Work out the finished part from the listing and answer in its coordinate system (mm). Face numbers are marked on the shaded views. A direction names the side the tool comes from. Give positions to 0.01 mm unless a question says otherwise; leave off trailing zeros. Loops run counter-clockwise (first coordinate to the right, second up) from the corner with the lowest first, then second, coordinate; pieces in that order, holes last. Notation, with made-up numbers: M 41,86 L 100,86 A19 ccw 100,102 Z; hole C 33.25,63 d8. An arc over 180 degrees is marked long. Use a Markdown table: item, result.
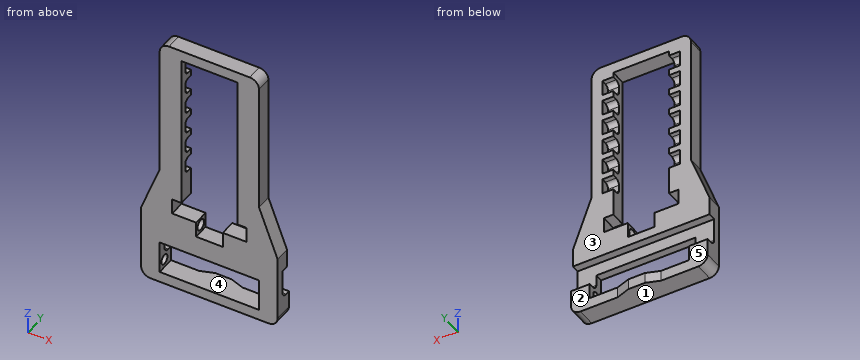
```python
from build123d import *
from OCP.BRepFilletAPI import BRepFilletAPI_MakeChamfer

# Parameters (mm, degrees)
SKETCH1_W                = 44
SKETCH1_H                = 22
BOSS_EXTRUDE1_DEPTH      = 5
SKETCH2_W                = 3.531949687
SKETCH2_H                = 41.5
SKETCH2_W_2              = 3.5
BOSS_EXTRUDE2_DEPTH      = 2
SKETCH3_W                = 44
SKETCH3_H                = 9.5
CUT_EXTRUDE1_DEPTH       = 2.5
SKETCH4_W                = 17.968050313
SKETCH4_H                = 14
CUT_EXTRUDE2_DEPTH       = 5
SKETCH5_W                = 24
SKETCH5_H                = 5
CUT_EXTRUDE3_DEPTH       = 5
SKETCH6_W                = 8.6
SKETCH6_H                = 5
CUT_EXTRUDE4_DEPTH       = 5
SKETCH7_W                = 14
SKETCH7_H                = 2
BOSS_EXTRUDE3_DEPTH      = 1.5
CHAMFER1_SIZE            = 1.5
CHAMFER1_SIZE_2          = 4.356316317
SKETCH8_W                = 32
SKETCH8_H                = 10
CUT_EXTRUDE5_DEPTH       = 5
FILLET3_R                = 3
SKETCH9_R                = 1.75
CUT_EXTRUDE6_DEPTH       = 3
CUT_EXTRUDE7_START       = -3
SKETCH10_R               = 1.75
CUT_EXTRUDE7_DEPTH       = 3
SKETCH11_R               = 1.6
CUT_EXTRUDE8_DEPTH       = 3
CUT_EXTRUDE9_START       = -3
SKETCH12_R               = 1.6
CUT_EXTRUDE9_DEPTH       = 3
SKETCH13_W               = 3.531949687
SKETCH13_H               = 2
BOSS_EXTRUDE5_DEPTH      = 3
FILLET4_R                = 1.5
BOSS_EXTRUDE6_DEPTH      = 2
BOSS_EXTRUDE6_DEPTH_BACK = 2
SKETCH15_W               = 6
SKETCH15_H               = 1
BOSS_EXTRUDE7_DEPTH      = 4.5
FILLET5_R                = 2
FILLET6_R                = 3
CUT_EXTRUDE10_DEPTH      = 14.5
CUT_EXTRUDE10_DEPTH_BACK = 14.5
SKETCH16_W               = 32
SKETCH16_H               = 0.5


with BuildPart() as part:
    # Sketch1 → Boss-Extrude1 (new body)
    with BuildSketch(Plane(origin=(0, 0, 0), x_dir=(1, 0, 0), z_dir=(0, 1, 0))):
        with Locations((0, 9)):
            Rectangle(SKETCH1_W, SKETCH1_H)
        Polygon((-16, -18), (16, -18), (22, -2), (-22, -2), align=None)
        Polygon((-12.5, -18), (-16, -18), (-16, -63), (16, -63), (16, -18), (12.5, -18), (12.5, -59.5), (-12.5, -59.5), align=None)
    extrude(amount=BOSS_EXTRUDE1_DEPTH)

    # Sketch2 → Boss-Extrude2 (add)
    with BuildSketch(Plane.XZ):
        with Locations((-10.734025156, 38.75)):
            Rectangle(SKETCH2_W, SKETCH2_H)
        with Locations((10.75, 38.75)):
            Rectangle(SKETCH2_W_2, SKETCH2_H)
    extrude(amount=-BOSS_EXTRUDE2_DEPTH)

    # Sketch3 → Cut-Extrude1 (cut)
    with BuildSketch(Plane(origin=(0, 5, 0), x_dir=(1, 0, 0), z_dir=(0, 1, 0))):
        with Locations((0, 8.75)):
            Rectangle(SKETCH3_W, SKETCH3_H)
    extrude(amount=-CUT_EXTRUDE1_DEPTH, mode=Mode.SUBTRACT)

    # Sketch4 → Cut-Extrude2 (cut)
    with BuildSketch(Plane(origin=(0, 5, 0), x_dir=(1, 0, 0), z_dir=(0, 1, 0))):
        with Locations((0.015974843, -11)):
            Rectangle(SKETCH4_W, SKETCH4_H)
    extrude(amount=-CUT_EXTRUDE2_DEPTH, mode=Mode.SUBTRACT)

    # Sketch5 → Cut-Extrude3 (cut)
    with BuildSketch(Plane(origin=(0, 5, 0), x_dir=(1, 0, 0), z_dir=(0, 1, 0))):
        with Locations((0.031949687, -6.5)):
            Rectangle(SKETCH5_W, SKETCH5_H)
    extrude(amount=-CUT_EXTRUDE3_DEPTH, mode=Mode.SUBTRACT)

    # Sketch6 → Cut-Extrude4 (cut)
    with BuildSketch(Plane(origin=(0, 5, 0), x_dir=(1, 0, 0), z_dir=(0, 1, 0))):
        with Locations((0.031949687, -1.5)):
            Rectangle(SKETCH6_W, SKETCH6_H)
    extrude(amount=-CUT_EXTRUDE4_DEPTH, mode=Mode.SUBTRACT)

    # Sketch7 → Boss-Extrude3 (add)
    with BuildSketch(Plane(origin=(0, 5, 0), x_dir=(1, 0, 0), z_dir=(0, 1, 0))):
        with Locations((0, 19)):
            Rectangle(SKETCH7_W, SKETCH7_H)
    extrude(amount=BOSS_EXTRUDE3_DEPTH)

    # Chamfer1
    chamfer1_edges_1 = [part.edges().sort_by_distance(p)[0] for p in [
        (7, 6.5, -19),
    ]]
    chamfer1_side_1 = [part.faces().sort_by_distance(p)[0] for p in [
        (7, 6.47, -19),
    ]]
    chamfer1_edges_2 = [part.edges().sort_by_distance(p)[0] for p in [
        (-7, 6.5, -19),
    ]]
    chamfer1_side_2 = [part.faces().sort_by_distance(p)[0] for p in [
        (-7, 6.47, -19),
    ]]
    chamfer1 = BRepFilletAPI_MakeChamfer(part.part.solid().wrapped)
    for e in chamfer1_edges_1:
        chamfer1.Add(CHAMFER1_SIZE - 0.0001, CHAMFER1_SIZE_2 - 0.0001, e.wrapped, chamfer1_side_1[0].wrapped)
    for e in chamfer1_edges_2:
        chamfer1.Add(CHAMFER1_SIZE - 0.0001, CHAMFER1_SIZE_2 - 0.0001, e.wrapped, chamfer1_side_2[0].wrapped)
    add(Compound.cast(chamfer1.Shape()), mode=Mode.REPLACE)  # a hair under: the kernel refuses the full size

    # Sketch8 → Cut-Extrude5 (cut)
    with BuildSketch(Plane(origin=(0, 5, 0), x_dir=(1, 0, 0), z_dir=(0, 1, 0))):
        with Locations((0, 13)):
            Rectangle(SKETCH8_W, SKETCH8_H)
    extrude(amount=-CUT_EXTRUDE5_DEPTH, mode=Mode.SUBTRACT)

    # Fillet3
    fillet3_edges = [part.edges().sort_by_distance(p)[0] for p in [
        (16, 2.5, 63),
        (-16, 2.5, 63),
    ]]
    fillet(fillet3_edges, radius=FILLET3_R)

    # Sketch9 → Cut-Extrude6 (cut)
    with BuildSketch(Plane(origin=(-4.268050313, 0, 0), x_dir=(0, 0, -1), z_dir=(1, 0, 0))):
        with Locations((-1.5, 2.5)):
            Circle(SKETCH9_R)
    extrude(amount=-CUT_EXTRUDE6_DEPTH, mode=Mode.SUBTRACT)

    # Sketch10 → Cut-Extrude7 (cut)
    with BuildSketch(Plane.ZY.offset(-4.331949687).offset(CUT_EXTRUDE7_START)):
        with Locations(Location((1.5, 2.5, 0), (0, 0, 180))):
            Circle(SKETCH10_R)
    extrude(amount=CUT_EXTRUDE7_DEPTH, mode=Mode.SUBTRACT)

    # Sketch11 → Cut-Extrude8 (cut)
    with BuildSketch(Plane.ZY.offset(-16)):
        with Locations((-15.75, 2.5)):
            Circle(SKETCH11_R)
    extrude(amount=-CUT_EXTRUDE8_DEPTH, mode=Mode.SUBTRACT)

    # Sketch12 → Cut-Extrude9 (cut)
    with BuildSketch(Plane(origin=(-16, 0, 0), x_dir=(0, 0, -1), z_dir=(1, 0, 0)).offset(CUT_EXTRUDE9_START)):
        with Locations(Location((15.75, 2.5, 0), (0, 0, 180))):
            Circle(SKETCH12_R)
    extrude(amount=CUT_EXTRUDE9_DEPTH, mode=Mode.SUBTRACT)

    # Sketch13 → Boss-Extrude5 (add)
    with BuildSketch(Plane(origin=(0, 2, 0), x_dir=(1, 0, 0), z_dir=(0, 1, 0))):
        with Locations((-10.734025156, -24)):
            Rectangle(SKETCH13_W, SKETCH13_H)
        with Locations((10.765974844, -24)):
            Rectangle(SKETCH13_W, SKETCH13_H)
        with Locations((10.765974844, -31)):
            Rectangle(SKETCH13_W, SKETCH13_H)
        with Locations((10.765974844, -38)):
            Rectangle(SKETCH13_W, SKETCH13_H)
        with Locations((10.765974844, -45)):
            Rectangle(SKETCH13_W, SKETCH13_H)
        with Locations((10.765974844, -52)):
            Rectangle(SKETCH13_W, SKETCH13_H)
        with Locations((10.765974844, -59)):
            Rectangle(SKETCH13_W, SKETCH13_H)
        with Locations((-10.734025156, -31)):
            Rectangle(SKETCH13_W, SKETCH13_H)
        with Locations((-10.734025156, -38)):
            Rectangle(SKETCH13_W, SKETCH13_H)
        with Locations((-10.734025156, -45)):
            Rectangle(SKETCH13_W, SKETCH13_H)
        with Locations((-10.734025156, -52)):
            Rectangle(SKETCH13_W, SKETCH13_H)
        with Locations((-10.734025156, -59)):
            Rectangle(SKETCH13_W, SKETCH13_H)
    extrude(amount=BOSS_EXTRUDE5_DEPTH)

    # Fillet4
    fillet4_edges = [part.edges().sort_by_distance(p)[0] for p in [
        (-10.734025157, 2, 23),
        (-10.734025157, 2, 25),
        (10.75, 2, 23),
        (10.75, 2, 25),
        (10.75, 2, 30),
        (10.75, 2, 32),
        (10.75, 2, 37),
        (10.75, 2, 39),
        (10.75, 2, 44),
        (10.75, 2, 46),
        (10.75, 2, 51),
        (10.75, 2, 53),
        (10.75, 2, 58),
        (-10.734025157, 2, 30),
        (-10.734025157, 2, 32),
        (-10.734025157, 2, 37),
        (-10.734025157, 2, 39),
        (-10.734025157, 2, 44),
        (-10.734025157, 2, 46),
        (-10.734025157, 2, 51),
        (-10.734025157, 2, 53),
        (-10.734025157, 2, 58),
        (-10.734025157, 2, 18),
        (10.75, 2, 18),
    ]]
    fillet(fillet4_edges, radius=FILLET4_R)

    # Sketch14 → Boss-Extrude6 (add, two sides: drawn at the far end of the back side and taken through both)
    with BuildSketch(Plane(origin=(0, 0, -20), x_dir=(-1, 0, 0), z_dir=(0, 0, -1)).offset(-BOSS_EXTRUDE6_DEPTH_BACK)):
        Polygon((-22, 6), (-22, 0), (22, 0), (22, 6), (7, 6), (2.643683683, 7.5), (-2.643683683, 7.5), (-7, 6), align=None)
    extrude(amount=BOSS_EXTRUDE6_DEPTH + BOSS_EXTRUDE6_DEPTH_BACK)

    # Sketch15 → Boss-Extrude7 (add)
    with BuildSketch(Plane.XY.offset(-18)):
        with Locations((19, 5.5)):
            Rectangle(SKETCH15_W, SKETCH15_H)
        with Locations((-19, 5.5)):
            Rectangle(SKETCH15_W, SKETCH15_H)
    extrude(amount=BOSS_EXTRUDE7_DEPTH)

    # Fillet5
    fillet5_edges = [part.edges().sort_by_distance(p)[0] for p in [
        (-19, 2.5, -13.5),
        (19, 2.5, -13.5),
    ]]
    fillet(fillet5_edges, radius=FILLET5_R)

    # Fillet6
    fillet6_edges = [part.edges().sort_by_distance(p)[0] for p in [
        (22, 3, -22),
        (-22, 3, -22),
    ]]
    fillet(fillet6_edges, radius=FILLET6_R)

    # Sketch16 → Cut-Extrude10 (cut, two sides: drawn at the far end of the back side and taken through both)
    with BuildSketch(Plane(origin=(0, 6, 0), x_dir=(1, 0, 0), z_dir=(0, 1, 0)).offset(-CUT_EXTRUDE10_DEPTH_BACK)):
        with Locations((0, 18.25)):
            Rectangle(SKETCH16_W, SKETCH16_H)
    extrude(amount=CUT_EXTRUDE10_DEPTH + CUT_EXTRUDE10_DEPTH_BACK, mode=Mode.SUBTRACT)


solid = part.part
```
(1) A cutting plane is placed at A-A (z = -15.75). Write down the section's boundary in (x, y), and give its area (3 significant figures).
Entries:
| item | result |
|---|---|
| outline | M -22,0 L -16,0 L -16,0.9 L -19,0.9 L -19,4.1 L -16,4.1 L -16,6 L -22,6 Z; M 16,0 L 22,0 L 22,6 L 16,6 L 16,4.1 L 19,4.1 L 19,0.9 L 16,0.9 Z |
| area | 52.8 mm² |
(2) A cutting plane is placed at C-C (x = 15). Write down the section's boundary in (y, z), and give its area (3 significant figures).
Entries:
| item | result |
|---|---|
| outline | M 0,-22 L 6,-22 L 6,-18.5 L 0,-18.5 Z; M 0,-8 L 2.5,-8 L 2.5,-4 L 5,-4 L 5,62.24 L 0,62.24 Z |
| area | 362 mm² |
(3) Which of the six approach directions +Z, -Z, +X, -X, +Y, -Y give full straight-line access (tool end or side, diameter ignored) to the marked faces 1, 2 and 3?
Entries:
| item | result |
|---|---|
| face 1 | -Z, +X, -X, +Y, -Y |
| face 2 | +Z, -Z, +X, +Y |
| face 3 | +Z, +X, -X, +Y |
(4) A cutting plane is placed at B-B (x = -17). Write down the section's boundary in (y, z), and give its area (3 significant figures).
Entries:
| item | result |
|---|---|
| outline | M 0,-22 L 6,-22 L 6,-13.5 L 4.5,-13.5 A2 cw 2.5,-11.5 L 2.5,-4 L 5,-4 L 5,15.33 L 0,15.33 Z; hole C 2.5,-15.75 d3.2 |
| area | 164 mm² |
(5) The mould has two halves that part along X. Classify the marked faces 4 and 5: released by +X, released by -X, zero draft, split by the parting line, or undercut.
Entries:
| item | result |
|---|---|
| face 4 | undercut |
| face 5 | zero draft |
(6) A cutting plane is placed at D-D (z = 15). Write down the section's boundary in (x, y) (3 decimals), and give its area (3 significant figures).
Entries:
| item | result |
|---|---|
| outline | M -17.125,0 L -8.968,0 L -8.968,5 L -17.125,5 Z; M 9,0 L 17.125,0 L 17.125,5 L 9,5 Z |
| area | 81.4 mm² |
(7) Consider probe 1 along Z at (x, y) = (2, 4.5); probe 2 along Y at (x, z) = (16.7, -15.75); probe 3 along Z at (x, y) = (-7, 1). Determine where each line is inside the solid, lowest interval first. Write a range as [from, to].
Entries:
| item | result |
|---|---|
| probe 1 | z = [-22, -18.5], [-4, -1], [59.5, 63] |
| probe 2 | y = [0, 0.9], [4.1, 6] |
| probe 3 | z = [-22, -18.5], [-8, 0.6], [2.4, 4], [59.5, 63] |
(8) Given P1, Ø1, axis at y = 3.5, z = 14, coming from the -X side; P2, Ø1, axis at x = 10, z = 35, coming from the +Y side; P3, Ø10, axis at x = -8.5, z = 34.5, coming from the +Y side, each flat-ended and moving along its own axis, determine where each tip first touches the part or whether it passes through.
Entries:
| item | result |
|---|---|
| P1 | stops at x = -17.69 |
| P2 | stops at y = 2 |
| P3 | stops at y = 5 |
